```python
from build123d import *

# Parameters (mm, degrees)
SKETCH_1_W          = 180
SKETCH_1_H          = 28
EXTRUDE_1_DEPTH     = 90
SKETCH_2_R          = 6
CUT_EXTRUDE_1_DEPTH = 30
SKETCH_3_W          = 180
SKETCH_3_H          = 60
CUT_EXTRUDE_2_DEPTH = 10


with BuildPart() as part:
    # 草图1 → 拉伸1 (new body)
    with BuildSketch(Plane.XY):
        with Locations((90, -14)):
            Rectangle(SKETCH_1_W, SKETCH_1_H)
    extrude(amount=EXTRUDE_1_DEPTH)

    # 草图2 → 切除-拉伸1 (cut)
    with BuildSketch(Plane.XY.offset(90)):
        with Locations((33, -14)):
            Circle(SKETCH_2_R)
        with Locations(Location((147, -14, 0), (0, 0, 180))):
            Circle(SKETCH_2_R)
    extrude(amount=-CUT_EXTRUDE_1_DEPTH, mode=Mode.SUBTRACT)

    # 草图3 → 切除-拉伸2 (cut)
    with BuildSketch(Plane(origin=(0, 0, 0), x_dir=(1, 0, 0), z_dir=(0, 1, 0))):
        with Locations((90, -30)):
            Rectangle(SKETCH_3_W, SKETCH_3_H)
    extrude(amount=-CUT_EXTRUDE_2_DEPTH, mode=Mode.SUBTRACT)


solid = part.part
```
The model under review builds one solid part; all positions refer to its coordinate system, in mm. A direction names the side the tool comes from. Round coordinates to 2 decimals unless told otherwise and drop trailing zeros. Loops run counter-clockwise (first coordinate to the right, second up) from the corner with the lowest first, then second, coordinate; pieces in that order, holes last. Notation, with made-up numbers: (84.25, -11) - (105.25, -11) arc R21 cw to (105.25, -5) - close; hole circle Ø3 at (36, 89.25). An arc over 180 degrees is marked (long way). Use a Markdown table: item, result. Add a question column.
Q1. Add section C-C (x = 13.5). State the section outline as (y, z) points.
Q2. Add section B-B (y = -12.25). State the section outline as (x, z) points.
Q3. Insertion check: pin 1 Ø18 at (x, z) = (126, 36) entering from +Y; pin 2 Ø11 at (x, y) = (147, -14) entering from +Z. Each pin has a flat end and moves straight along its axis. Give the tip position at first contact, or say it passes through.
Q4. For probe 1 along X at (y, z) = (-14, 66.5); probe 2 along Y at (x, z) = (33, 80.75); probe 3 along X at (y, z) = (-11.5, 67), list the stretches that pass through material, from the lowest coordinate up.
Q5. Add section D-D (z = 28). State the section outline as (x, y) points, plus the area to 3 significant figures.
Q6. Machinability: for faces 1 (the face through (89, -19, 0)), 2 (the face through (89, -5, 60)), 3 (the face through (33, -15, 60)), which of the approach directions +Z, -Z, +X, -X, +Y, -Y give a long, thin tool a straight path to every point of the face, cutting with its end or side? Answer none if there is none.
Q7. The part is to be moulded in two halves that separate along Y. For faces 4 (the face through (28.58, -9.94, 75.21)), 5 (the face through (89, -14, 90)), 6 (the face through (89, -28, 44)), 7 (the face through (147, -15, 60)), say which applies: pulls with the +Y half, pulls with the -Y half, needs draft (parallel to the pull), parting line crosses it, or undercut.
Q8. Add section A-A (x = 147). State the section outline as (y, z) points.
Worked answers:
| question | item | result |
|---|---|---|
| 1 | outline | (-28, 0) - (-10, 0) - (-10, 60) - (0, 60) - (0, 90) - (-28, 90) - close |
| 2 | outline | (0, 0) - (180, 0) - (180, 90) - (152.74, 90) - (152.74, 60) - (141.26, 60) - (141.26, 90) - (38.74, 90) - (38.74, 60) - (27.26, 60) - (27.26, 90) - (0, 90) - close |
| 3 | pin 1 | y = -10 |
| 3 | pin 2 | z = 60 |
| 4 | probe 1 | 0 to 27, 39 to 141, 153 to 180 |
| 4 | probe 2 | -28 to -20, -8 to 0 |
| 4 | probe 3 | 0 to 27.55, 38.45 to 141.55, 152.45 to 180 |
| 5 | outline | (0, -28) - (180, -28) - (180, -10) - (0, -10) - close |
| 5 | area | 3,240 mm² |
| 6 | face 1 | -Z, +X, -X, +Y, -Y |
| 6 | face 2 | -Z, +X, -X, +Y |
| 6 | face 3 | +Z |
| 7 | face 4 | undercut |
| 7 | face 5 | needs draft |
| 7 | face 6 | pulls with the -Y half |
| 7 | face 7 | undercut |
| 8 | outline | (-28, 0) - (-10, 0) - (-10, 60) - (-20, 60) - (-20, 90) - (-28, 90) - close; (-8, 60) - (0, 60) - (0, 90) - (-8, 90) - close |
